Check sheet for the modelled part. Datum: model origin and axes. Units: mm. A direction names the side the tool comes from. Give positions to 0.01 mm unless a question says otherwise; leave off trailing zeros. Write each loop counter-clockwise with the first axis right and the second up, starting at its lowest first coordinate (ties: lowest second). Pieces come first, ordered by that corner, then holes. Notation, with made-up numbers: (64, 44.25) -> (114, 44.25) arc R14 cw to (114, 49.25) -> close; hole circle Ø5 at (22.25, 80.25). An arc over 180 degrees is marked (long way). Return JSON: item names as keys, results as strings.
from build123d import *

# Parameters (mm, degrees)
BLANKSKE_W         = 170
BLANKSKE_H         = 33.5
BLANK_DEPTH        = 20
TOOTHCUTSIM_DEPTH  = 175.419752322
TEETHCUTS_COUNT    = 16
TEETHCUTS_PITCH    = 10.995574275
SKETCH2_W          = 9
SKETCH2_H          = 4
CUT_EXTRUDE1_DEPTH = 15
SKETCH4_R          = 2.75
CUT_EXTRUDE2_DEPTH = 20


with BuildPart() as part:
    # BlankSke → Blank (new body)
    with BuildSketch(Plane.XY):
        with Locations((85, 16.75)):
            Rectangle(BLANKSKE_W, BLANKSKE_H)
    extrude(amount=-BLANK_DEPTH)

    # TooCutSkeSim → ToothCutSim (cut, through all)
    with BuildSketch(Plane.XY):
        Polygon((1.507523794, 25.625), (-1.507523794, 25.625), (-4.383034233, 33.5254), (4.383034233, 33.5254), align=None)
    toothcutsim = extrude(amount=-TOOTHCUTSIM_DEPTH, mode=Mode.SUBTRACT)

    # TeethCuts: ToothCutSim ×16
    with Locations(*[(i * TEETHCUTS_PITCH, 0, 0) for i in range(1, TEETHCUTS_COUNT)]):
        add(toothcutsim, mode=Mode.SUBTRACT)

    # Sketch2 → Cut-Extrude1 (cut)
    with BuildSketch(Plane.XY):
        with Locations((15, 12)):
            Rectangle(SKETCH2_W, SKETCH2_H)
        with Locations((43, 12)):
            Rectangle(SKETCH2_W, SKETCH2_H)
        with Locations((133, 12)):
            Rectangle(SKETCH2_W, SKETCH2_H)
        with Locations((159, 12)):
            Rectangle(SKETCH2_W, SKETCH2_H)
    extrude(amount=-CUT_EXTRUDE1_DEPTH, mode=Mode.SUBTRACT)

    # Sketch4 → Cut-Extrude2 (cut)
    with BuildSketch(Plane.XZ):
        with Locations(Location((15, -5, 0), (0, 0, 270))):
            Circle(SKETCH4_R)
        with Locations(Location((43, -5, 0), (0, 0, 270))):
            Circle(SKETCH4_R)
        with Locations(Location((133, -5, 0), (0, 0, 270))):
            Circle(SKETCH4_R)
        with Locations(Location((159, -5, 0), (0, 0, 270))):
            Circle(SKETCH4_R)
    extrude(amount=-CUT_EXTRUDE2_DEPTH, mode=Mode.SUBTRACT)


solid = part.part
(1) Cross-section at B-B on z = -11. State how many separate pieces and enclosed holes the cut face has, then the cut area to 3 significant figures.
Reply:
{"separate pieces": "1", "enclosed holes": "4", "area": "4,830 mm^2"}
(2) Release check for a two-part mould opening along X. For faces 4 (the flat face through (90.925, 29.618, -9.86)), 5 (the flat face through (154, 25.625, -10)), 6 (the flat face through (0, 13, -10)) record: pulls with the +X half, pulls with the -X half, needs draft (parallel to the pull), parting line crosses it, or undercut.
Reply:
{"face 4": "undercut", "face 5": "undercut", "face 6": "pulls with the -X half"}
(3) Set-up check for faces 1 (the flat face through (46.943, 29.618, -9.86)), 2 (the flat face through (133, 14, -9)), 3 (the cylindrical face through (17.727, 4.93, -4.642)): record each of +Z, -Z, +X, -X, +Y, -Y from which the full face is reachable in a straight line by a thin tool's end or side.
Reply:
{"face 1": "+Z, -Z, +Y", "face 2": "+Z", "face 3": "-Y"}
(4) Depth check by flat-ended pin: pin 1 Ø0.9 at (x, z) = (76.5, -6) entering from +Y (3 decimals); pin 2 Ø3 at (x, z) = (44, -5.5) entering from -Y. Enter the tip coordinate at first touch or a pass-through.
Reply:
{"pin 1": "y = 25.625", "pin 2": "y = 20"}
(5) Thickness scan on L1, parallel to X at y = 4.5, z = -5; L2, parallel to Z at x = 159, y = 17; L3, parallel to X at y = 6, z = -2.75. Record the ranges inside material, lowest first.
Reply:
{"L1": "0 to 12.25, 17.75 to 40.25, 45.75 to 130.25, 135.75 to 156.25, 161.75 to 170", "L2": "-20 to -7.75, -2.25 to 0", "L3": "0 to 13.42, 16.58 to 41.42, 44.58 to 131.42, 134.58 to 157.42, 160.58 to 170"}
(6) Cross-section at A-A on y = 3.5. Enter the section's corners in (x, z), then the cut area to 3 significant figures.
Reply:
{"outline": "(0, -20) -> (170, -20) -> (170, 0) -> (0, 0) -> close; hole circle Ø5.5 at (15, -5); hole circle Ø5.5 at (43, -5); hole circle Ø5.5 at (133, -5); hole circle Ø5.5 at (159, -5)", "area": "3,300 mm^2"}
